Geometry check sheet. Reference: drawing and pictorial views, mm from the part's lowest x, y, z. A direction names the side the tool comes from. Round coordinates to 2 decimals unless told otherwise and drop trailing zeros. Loops run counter-clockwise (first coordinate to the right, second up) from the corner with the lowest first, then second, coordinate; pieces in that order, holes last. Notation, with made-up numbers: (-30.5, 88.25) -> (-13.5, 88.25) arc R20 ccw to (-13.5, 116.25) -> close; hole circle Ø3 at (10.5, -35). An arc over 180 degrees is marked (long way). Write item = value, one per line.
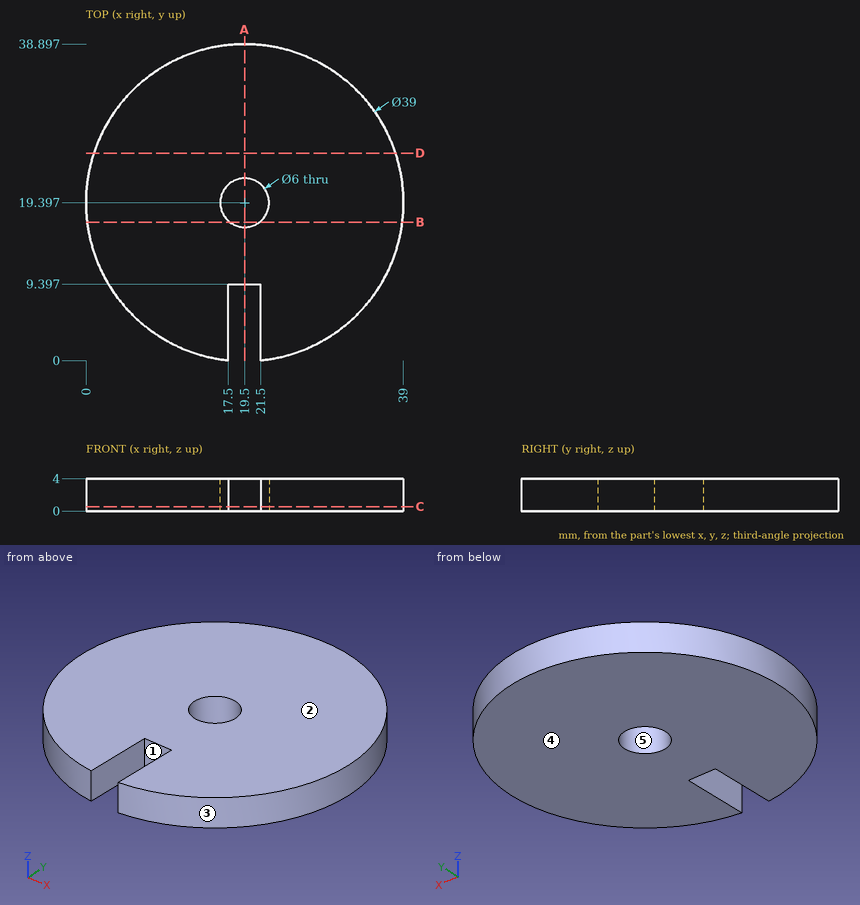
(1) Set-up check for the marked faces 1 and 2: record each of +Z, -Z, +X, -X, +Y, -Y from which the full face is reachable in a straight line by a thin tool's end or side.
Filled sheet:
face_1 = +Z, -Z, -Y
face_2 = +Z, +X, -X, +Y, -Y
(2) Sectioned sample at C-C, the plane z = 0.55. Record the cut outline in (x, y).
Filled sheet:
outline = (17.5, 0) -> (17.5, 9.4) -> (21.5, 9.4) -> (21.5, 0) arc R19.5 ccw (long way) to start; hole circle Ø6 at (19.5, 19.4)
(3) Sectioned sample at D-D, the plane y = 25.5. Record the cut outline in (x, z).
Filled sheet:
outline = (0.98, 0) -> (38.02, 0) -> (38.02, 4) -> (0.98, 4) -> close
(4) Sectioned sample at B-B, the plane y = 17. Record the cut outline in (x, z), and give its area (3 significant figures).
Filled sheet:
outline = (0.15, 0) -> (17.7, 0) -> (17.7, 4) -> (0.15, 4) -> close; (21.3, 0) -> (38.85, 0) -> (38.85, 4) -> (21.3, 4) -> close
area = 140 mm2
(5) Draft check along X on the marked faces 3, 4 and 5. Enter one of: released by +X, released by -X, zero draft, split by the parting line, or undercut.
Filled sheet:
face_3 = split by the parting line
face_4 = zero draft
face_5 = undercut
(6) Sectioned sample at A-A, the plane x = 19.5. Record the cut outline in (y, z).
Filled sheet:
outline = (9.4, 0) -> (16.4, 0) -> (16.4, 4) -> (9.4, 4) -> close; (22.4, 0) -> (38.9, 0) -> (38.9, 4) -> (22.4, 4) -> close
(7) Go/stop test with flat-tipped pins: pin 1 Ø2 at (y, z) = (6.5, 2) entering from +X; pin 2 Ø1.2 at (x, z) = (20, 2) entering from -Y; pin 3 Ø2 at (y, z) = (23, 1.5) entering from -X. Record where each tip stops, or that it passes through.
Filled sheet:
pin_1 = 34.95
pin_2 = 9.4
pin_3 = 0.17
(8) Material ranges on probe 1 along Y at (x, z) = (19.5, 1.4); probe 2 along X at (y, z) = (3, 2.7) (1 decimal); probe 3 along X at (y, z) = (20, 2.9), recorded low to high. Write a range as from..to.
Filled sheet:
probe_1 = 9.4..16.4, 22.4..38.9
probe_2 = 8.9..17.5, 21.5..30.1
probe_3 = 0.01..16.56, 22.44..38.99
